Input: part model. Units: mm. Frame: model coordinates. Round coordinates to 2 decimals unless told otherwise and drop trailing zeros. Write each loop counter-clockwise with the first axis right and the second up, starting at its lowest first coordinate (ties: lowest second). Pieces come first, ordered by that corner, then holes. Notation, with made-up numbers: (67.25, 73.25) -> (105.25, 73.25) arc R18 cw to (105.25, 105.25) -> close; hole circle Ø11 at (-5, 82.25). An arc over 180 degrees is marked (long way). Use CSV: the item, a comma, the result in double quotes.
```python
from build123d import *

# Parameters (mm, degrees)
SKETCH_1_R          = 10
EXTRUDE_1_DEPTH     = 25
SKETCH_3_R          = 4
CUT_EXTRUDE_1_DEPTH = 7.5
SKETCH_4_R          = 5
CUT_EXTRUDE_2_DEPTH = 12.5
SKETCH_5_R          = 4
CUT_EXTRUDE_3_DEPTH = 23.5


with BuildPart() as part:
    # 草图1 → 凸台-拉伸1 (new body)
    with BuildSketch(Plane.XY):
        Circle(SKETCH_1_R)
    extrude(amount=EXTRUDE_1_DEPTH)

    # 草图3 → 切除-拉伸1 (cut)
    with BuildSketch(Plane.XY.offset(25)):
        Circle(SKETCH_3_R)
    extrude(amount=-CUT_EXTRUDE_1_DEPTH, mode=Mode.SUBTRACT)

    # 草图4 → 切除-拉伸2 (cut)
    with BuildSketch(Plane(origin=(0, 0, 0), x_dir=(-1, 0, 0), z_dir=(0, 0, -1))):
        Circle(SKETCH_4_R)
    extrude(amount=-CUT_EXTRUDE_2_DEPTH, mode=Mode.SUBTRACT)

    # 草图5 → 切除-拉伸3 (cut, through all)
    with BuildSketch(Plane.XY.offset(17.5)):
        Circle(SKETCH_5_R)
    extrude(amount=-CUT_EXTRUDE_3_DEPTH, mode=Mode.SUBTRACT)


solid = part.part
```
Item 1: Section query A-A on x = 0. Return the cut outline in (y, z), plus the area to 3 significant figures.
Worked answers:
outline,"(-10, 0) -> (-5, 0) -> (-5, 12.5) -> (-4, 12.5) -> (-4, 25) -> (-10, 25) -> close; (4, 12.5) -> (5, 12.5) -> (5, 0) -> (10, 0) -> (10, 25) -> (4, 25) -> close"
area,"275 mm²"
Item 2: Section query D-D on y = 8. Return the cut outline in (x, z), plus the area to 3 significant figures.
Worked answers:
outline,"(-6, 0) -> (6, 0) -> (6, 25) -> (-6, 25) -> close"
area,"300 mm²"
Item 3: First-contact query: pin 1 Ø12 at (x, z) = (6.5, 17.5) entering from +Y; pin 2 Ø1.5 at (x, y) = (-7.5, -6.5) entering from -Z; pin 3 Ø2 at (y, z) = (7.5, 22) entering from -X; pin 4 Ø1.5 at (y, z) = (-6, 19) entering from +X. Flat tips, straight axial feed; report the tip coordinate or a pass-through.
Worked answers:
pin 1,"stops at y = 9.99"
pin 2,"stops at z = 0"
pin 3,"stops at x = -7.6"
pin 4,"stops at x = 8.51"
Item 4: Line query: line 1 (Y direction, x = 0, z = 3.75); line 2 (Y direction, x = 0, z = 18); line 3 (X direction, y = 3, z = 22.5). Output: solid intervals per line, ascending.
Worked answers:
line 1,"y = -10 to -5, 5 to 10"
line 2,"y = -10 to -4, 4 to 10"
line 3,"x = -9.54 to -2.65, 2.65 to 9.54"
Item 5: Section query C-C on z = 10.75. Return the cut outline in (x, y), plus the area to 3 significant figures.
Worked answers:
outline,"circle Ø20 at (0, 0); hole circle Ø10 at (0, 0)"
area,"236 mm²"
Item 6: Pull-direction query (Y, two-part tool) for faces 1 (the face through (1.08, -4.88, 6.16)), 2 (the face through (-5, -2, 0)), 3 (the face through (-2.17, -9.76, 12.32)); classes: +Y half, -Y half, draft (parallel to the pull), parting line (faces both ways), or undercut.
Worked answers:
face 1,"undercut"
face 2,"draft"
face 3,"parting line"
